Verification items for the finished model (mm, model axes). A direction names the side the tool comes from. Coordinates: 2 decimals unless noted, no trailing zeros. Write each loop counter-clockwise with the first axis right and the second up, starting at its lowest first coordinate (ties: lowest second). Pieces come first, ordered by that corner, then holes. Notation, with made-up numbers: (46.25, 62.5) -> (90.25, 62.5) arc R15 cw to (90.25, 70.5) -> close; hole circle Ø2 at (-32, 26). An arc over 180 degrees is marked (long way). Answer in a Markdown table with one row per item.
```python
from build123d import *

# Parameters (mm, degrees)
F0_W        = 45
F0_H        = 50
F1_DEPTH    = 30
F2_W        = 40
F2_H        = 42
F3_DEPTH    = 30.001
F4_T1_DEPTH = 78.5477272148
F4_T3_DEPTH = 78.5477272148
F5_R        = 3.3798989873
F6_SIZE     = 5
F7_R        = 1.0624158
F7_R_2      = 1.974265
F8_DEPTH    = 45.001


# Not quite as in the source:
# - a fillet or chamfer that OpenCascade refuses, or shapes differently, is made with other operations: its cross-section is extruded or revolved along the edge and cut away or added


with BuildPart() as f1:
    # F0 (on Front) → F1 (new body)
    with BuildSketch(Plane.XZ):
        with Locations((5.6927716359, 6.5557161967)):
            Rectangle(F0_W, F0_H)
    extrude(amount=F1_DEPTH)

    # F2 (on face) → F3 (cut, through all)
    with BuildSketch(Plane.XZ.offset(30)):
        with Locations((5.6927716359, 10.5557161967)):
            Rectangle(F2_W, F2_H)
    extrude(amount=-F3_DEPTH, mode=Mode.SUBTRACT)

    # F4: fillet of radius 15.209545443 on 4 edges, made by hand

    # F4_s2 → F4_t1 (cut)
    with BuildSketch(Plane.YZ.offset(-54.8310919714)):
        with BuildLine():
            ThreePointArc((0, 16.3461707538), (-4.4547727215, 27.1009434752), (-15.209545443, 31.5557161967))
            Line((-15.209545443, 31.5557161967), (0, 31.5557161967))
            Line((0, 31.5557161967), (0, 16.3461707538))
        make_face()
        with BuildLine():
            ThreePointArc((-30, 16.3461707538), (-25.5452272785, 27.1009434752), (-14.790454557, 31.5557161967))
            Line((-14.790454557, 31.5557161967), (-30, 31.5557161967))
            Line((-30, 31.5557161967), (-30, 16.3461707538))
        make_face()
    extrude(amount=F4_T1_DEPTH, mode=Mode.SUBTRACT)

    # F4_s4 → F4_t3 (cut)
    with BuildSketch(Plane.YZ.offset(-12.3310919714)):
        with BuildLine():
            ThreePointArc((-14.790454557, 31.5557161967), (-25.5452272785, 27.1009434752), (-30, 16.3461707538))
            Line((-30, 16.3461707538), (-30, 31.5557161967))
            Line((-30, 31.5557161967), (-14.790454557, 31.5557161967))
        make_face()
        with BuildLine():
            ThreePointArc((-15.209545443, 31.5557161967), (-4.4547727215, 27.1009434752), (0, 16.3461707538))
            Line((0, 16.3461707538), (0, 31.5557161967))
            Line((0, 31.5557161967), (-15.209545443, 31.5557161967))
        make_face()
    extrude(amount=F4_T3_DEPTH, mode=Mode.SUBTRACT)

    # F5
    f5_edges = [f1.edges().sort_by_distance(p)[0] for p in [
        (-14.307228, -15, -10.444284),
        (25.692772, -15, -10.444284),
    ]]
    fillet(f5_edges, radius=F5_R)

    # F6
    f6_edges = [f1.edges().sort_by_distance(p)[0] for p in [
        (-16.807228, -15, -18.444284),
        (28.192772, -15, -18.444284),
    ]]
    chamfer(f6_edges, length=F6_SIZE)

    # F7 (on face) → F8 (cut, through all)
    with BuildSketch(Plane(origin=(-16.8072283641, 0, 0), x_dir=(0, -1, 0), z_dir=(-1, 0, 0))):
        with Locations((3.9704506522, 12.6322340244)):
            Circle(F7_R)
        with Locations((15.0680806522, 23.7298640244)):
            Circle(F7_R)
        with Locations((26.1657106522, 12.6322340244)):
            Circle(F7_R)
        with Locations((15.0680806522, 1.5346040244)):
            Circle(F7_R)
        with Locations((15.0680806522, 12.6322340244)):
            Circle(F7_R_2)
    extrude(amount=-F8_DEPTH, mode=Mode.SUBTRACT)


solid = f1.part
```
1. Sectioned sample at B-B, the plane y = -11. Record the cut outline in (x, z), and give its area (3 significant figures).
Findings below:
| item | result |
|---|---|
| outline | (-16.81, -13.44) -> (-11.81, -18.44) -> (23.19, -18.44) -> (28.19, -13.44) -> (28.19, 30.96) -> (25.69, 30.96) -> (25.69, -7.06) arc R3.38 cw to (22.31, -10.44) -> (-10.93, -10.44) arc R3.38 cw to (-14.31, -7.06) -> (-14.31, 30.96) -> (-16.81, 30.96) -> close |
| area | 547 mm² |
2. Sectioned sample at C-C, the plane x = 9. Record the cut outline in (y, z), and give its area (3 significant figures).
Findings below:
| item | result |
|---|---|
| outline | (-30, -18.44) -> (0, -18.44) -> (0, -10.44) -> (-30, -10.44) -> close |
| area | 240 mm² |
3. Material ranges on probe 1 along X at (y, z) = (-9.75, 21); probe 2 along Z at (x, y) = (3, -19.75); probe 3 along Z at (x, y) = (-13.5, -11), recorded low to high. Write a range as from..to.
Findings below:
| item | result |
|---|---|
| probe 1 | x = -16.81..-14.31, 25.69..28.19 |
| probe 2 | z = -18.44..-10.44 |
| probe 3 | z = -16.75..-9.26 |
4. Sectioned sample at A-A, the plane z = 7. Record the cut outline in (x, y), and give its area (3 significant figures).
Findings below:
| item | result |
|---|---|
| outline | (-16.81, -30) -> (-14.31, -30) -> (-14.31, 0) -> (-16.81, 0) -> close; (25.69, -30) -> (28.19, -30) -> (28.19, 0) -> (25.69, 0) -> close |
| area | 150 mm² |
5. Release check for a two-part mould opening along X. For faces 1 (the face through (-15.575, -4.265, 26.908)), 2 (the face through (-16.807, -15, 9)), 3 (the face through (25.693, -15, 8)) record: released by +X, released by -X, zero draft, split by the parting line, or undercut.
Findings below:
| item | result |
|---|---|
| face 1 | zero draft |
| face 2 | released by -X |
| face 3 | undercut |
6. Go/stop test with a flat-tipped pin: pin 1 (6 mm diameter, centred on x = 5.5, y = -23.5, fed in from +Z). Record where the tip stops, or that it passes through.
Findings below:
| item | result |
|---|---|
| pin 1 | stops at z = -10.44 |
7. Access from +Z, -Z, +X, -X, +Y, -Y to the whole of each face (thin tool, end or side, straight path). Record for faces 4 (the face through (-14.307, -15, 8)), 5 (the face through (26.925, -25.502, 27.144)).
Findings below:
| item | result |
|---|---|
| face 4 | +Z, +Y, -Y |
| face 5 | +Z, +X, -X, -Y |
8. Sectioned sample at D-D, the plane z = 21. Record the cut outline in (x, y), and give its area (3 significant figures).
Findings below:
| item | result |
|---|---|
| outline | (-16.81, -29.27) -> (-14.31, -29.27) -> (-14.31, -0.73) -> (-16.81, -0.73) -> close; (25.69, -29.27) -> (28.19, -29.27) -> (28.19, -0.73) -> (25.69, -0.73) -> close |
| area | 143 mm² |
